```python
from build123d import *

# Parameters (mm, degrees)
SKETCH1_W           = 32
SKETCH1_H           = 35
BOSS_EXTRUDE1_DEPTH = 2
M6_TAPPED_HOLE3_D   = 5
M6_TAPPED_HOLE4_D   = 5


with BuildPart() as part:
    # Sketch1 → Boss-Extrude1 (new body)
    with BuildSketch(Plane.XY):
        with Locations((1.67, -5.25)):
            Rectangle(SKETCH1_W, SKETCH1_H)
    extrude(amount=BOSS_EXTRUDE1_DEPTH)

    # M6 Tapped Hole3 (through all)
    with Locations(Plane(origin=(0, 0, 0), x_dir=(-1, 0, 0), z_dir=(0, 0, -1))):
        with Locations((9.83, -18.25), (-13.17, -18.25), (-13.17, 7.75), (9.83, 7.75)):
            Hole(M6_TAPPED_HOLE3_D / 2)

    # M6 Tapped Hole4 (through all)
    with Locations(Plane(origin=(0, 0, 0), x_dir=(-1, 0, 0), z_dir=(0, 0, -1))):
        with Locations((5.33, -5.25)):
            Hole(M6_TAPPED_HOLE4_D / 2)


solid = part.part
```
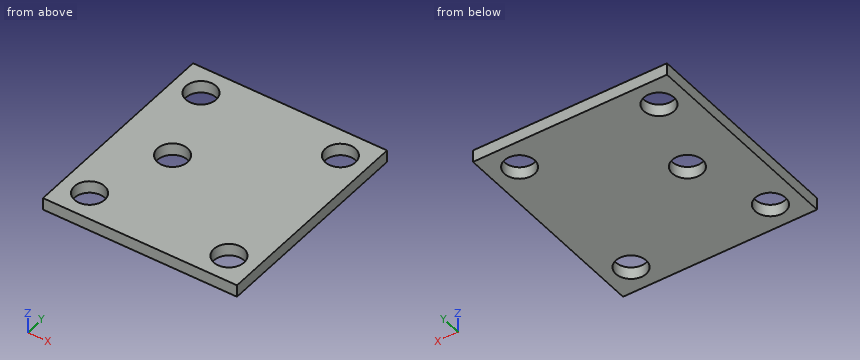
The listing builds one solid part. Answer for the finished solid, in the listing's coordinates (mm). Coordinates: 2 decimals unless noted, no trailing zeros. Loops run counter-clockwise (first coordinate to the right, second up) from the corner with the lowest first, then second, coordinate; pieces in that order, holes last. Notation, with made-up numbers: (0, -31.5) -> (58, -31.5) arc R15 ccw to (58, -13.5) -> close; hole circle Ø6 at (53, 75). An arc over 180 degrees is marked (long way). Return JSON: item names as keys, results as strings. Group by question number.
(1) A cutting plane is placed at A-A on x = -9.83. Write down the section's boundary in (y, z).
(2) A cutting plane is placed at B-B on y = 7.75. Write down the section's boundary in (x, z), and give its area (3 significant figures).
(3) A cutting plane is placed at C-C on y = -5.25. Write down the section's boundary in (x, z).
(4) Find the intervals of material crossed by probe 1 along Y at (x, z) = (13.17, 0.5); probe 2 along X at (y, z) = (-17, 0.35); probe 3 along X at (y, z) = (8, 0.3), in increasing order. Write a range as from..to.
The answers:
{
 "1": {"outline": "(-22.75, 0) -> (-20.75, 0) -> (-20.75, 2) -> (-22.75, 2) -> close; (-15.75, 0) -> (5.25, 0) -> (5.25, 2) -> (-15.75, 2) -> close; (10.25, 0) -> (12.25, 0) -> (12.25, 2) -> (10.25, 2) -> close"},
 "2": {"outline": "(-14.33, 0) -> (-12.33, 0) -> (-12.33, 2) -> (-14.33, 2) -> close; (-7.33, 0) -> (10.67, 0) -> (10.67, 2) -> (-7.33, 2) -> close; (15.67, 0) -> (17.67, 0) -> (17.67, 2) -> (15.67, 2) -> close", "area": "44.0 mm^2"},
 "3": {"outline": "(-14.33, 0) -> (-7.83, 0) -> (-7.83, 2) -> (-14.33, 2) -> close; (-2.83, 0) -> (17.67, 0) -> (17.67, 2) -> (-2.83, 2) -> close"},
 "4": {"probe 1": "y = -22.75..-20.75, -15.75..5.25, 10.25..12.25", "probe 2": "x = -14.33..-12, -7.66..11, 15.34..17.67", "probe 3": "x = -14.33..-12.32, -7.34..10.68, 15.66..17.67"}
}
